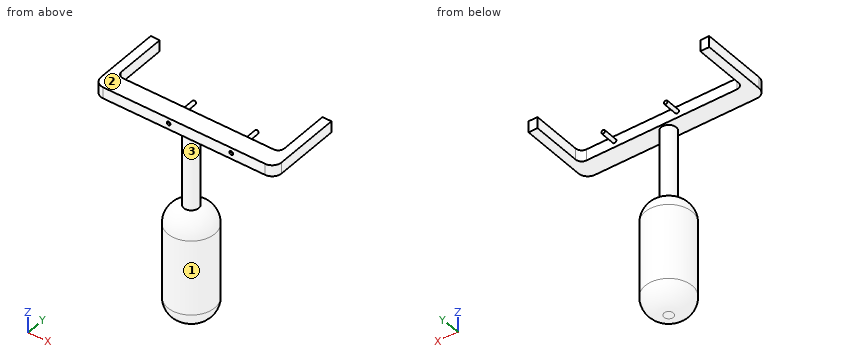
from build123d import *

# Parameters (mm, degrees)
F1_DEPTH  = 6
F2_R      = 3.25
F3_R      = 5
F4_R      = 1
F5_DEPTH  = 10
F6_R      = 4
F7_DEPTH  = 40
F8_R      = 12.5
F8_R_2    = 4
F9_DEPTH  = 60
F12_R     = 1
F13_DEPTH = 17


# Not quite as in the source:
# - a fillet or chamfer that OpenCascade refuses, or shapes differently, is made with other operations: its cross-section is extruded or revolved along the edge and cut away or added


with BuildPart() as f1:
    # F0 (on Top) → F1 (new body)
    with BuildSketch(Plane.XY):
        Polygon((-48, -5), (-48, -45), (48, -45), (48, -5), (43.25, -5), (43.25, -35), (-43.25, -35), (-43.25, -5), align=None)
    extrude(amount=F1_DEPTH)

    # F2
    f2_edges = [f1.edges().sort_by_distance(p)[0] for p in [
        (-43.25, -35, 3),
        (43.25, -35, 3),
    ]]
    fillet(f2_edges, radius=F2_R)

    # F3
    f3_edges = [f1.edges().sort_by_distance(p)[0] for p in [
        (48, -45, 3),
        (-48, -45, 3),
    ]]
    fillet(f3_edges, radius=F3_R)

    # F4 (on face) → F5 (cut)
    with BuildSketch(Plane.XZ.offset(45)):
        with Locations((-8.25, 3.2)):
            Circle(F4_R)
        with Locations((25, 3.2)):
            Circle(F4_R)
    extrude(amount=-F5_DEPTH, mode=Mode.SUBTRACT)

    # F6 (on face) → F7 (join)
    with BuildSketch(Plane(origin=(0, 0, 0), x_dir=(1, 0, 0), z_dir=(0, 0, -1))):
        with Locations((0, 40)):
            Circle(F6_R)
    extrude(amount=F7_DEPTH)

    # F8 (on face) → F9 (join)
    with BuildSketch(Plane(origin=(0, 0, -40), x_dir=(1, 0, 0), z_dir=(0, 0, -1))):
        with Locations((0, 40)):
            Circle(F8_R)
        with Locations((0, 40)):
            Circle(F8_R_2, mode=Mode.SUBTRACT)
        with Locations((0, 40)):
            Circle(F8_R_2)
    extrude(amount=F9_DEPTH)

    # F10: fillet of radius 10 on 2 edges, made by hand

    # F10_s1 → F10_t2 (revolve, cut)
    with BuildSketch(Plane.XZ.offset(40)):
        with BuildLine():
            ThreePointArc((12.5, -90), (9.5710678119, -97.0710678119), (2.5, -100))
            Line((2.5, -100), (12.5, -100))
            Line((12.5, -100), (12.5, -90))
        make_face()
    revolve(axis=Axis((0, -40, -100), (0, 0, -1)), mode=Mode.SUBTRACT)

    # F10_s3 → F10_t4 (revolve, cut)
    with BuildSketch(Plane.XZ.offset(40)):
        with BuildLine():
            ThreePointArc((12.5, -49.8868599666), (10.0828754441, -43.3676575614), (4, -40))
            Line((4, -40), (12.5, -40))
            Line((12.5, -40), (12.5, -49.8868599666))
        make_face()
    revolve(axis=Axis((0, -40, -40), (0, 0, -1)), mode=Mode.SUBTRACT)

    # F12 (on offset) → F13 (join)
    with BuildSketch(Plane.XZ.offset(44)):
        with Locations((-8.25, 3.2)):
            Circle(F12_R)
        with Locations((25, 3.2)):
            Circle(F12_R)
    extrude(amount=-F13_DEPTH)


solid = f1.part
Geometry check sheet. Reference: the model listing, model coordinates, mm. Face numbers are marked on the shaded views. Coordinates: 2 decimals unless noted, no trailing zeros. Order: outer loops, then holes, each group sorted by start corner. A loop starts at its lowest first (then second) coordinate and runs counter-clockwise, first axis right, second up. Notation, with made-up numbers: (62.5, 88.25) -> (104.5, 88.25) arc R17 ccw to (104.5, 97.25) -> close; hole circle Ø3 at (-17.5, -13.5). An arc over 180 degrees is marked (long way). Use a Markdown table: item, result. Add a question column.
1. Cross-section at A-A (y = -15). Enter the section's corners in (x, z).
2. Go/stop test with flat-tipped pins: pin 1 Ø0.6 at (x, z) = (-8, 3) entering from -Y; pin 2 Ø10 at (y, z) = (-25, -80.5) entering from +X; pin 3 Ø8 at (y, z) = (-45, -44) entering from +X; pin 4 Ø20 at (x, y) = (16.5, -16.5) entering from -Z. Record where each tip stops, or that it passes through.
3. Material ranges on L1, parallel to X at y = -14, z = 1; L2, parallel to X at y = -36.5, z = -12; L3, parallel to X at y = -35, z = -91.5, recorded low to high.
4. Mould release check, pull along Z, two halves, no side actions. Record for the marked faces 1, 2 and 3: pulls with the +Z half, pulls with the -Z half, needs draft (parallel to the pull), parting line crosses it, or undercut.
5. Cross-section at B-B (x = -14). Enter the section's corners in (y, z), and give its area (3 significant figures).
6. Cross-section at D-D (y = -30.5). Give the number of separate pieces and of enclosed holes in the cut face, and give its area (3 significant figures).
7. Cross-section at C-C (z = -22). Enter the section's corners in (x, y).
Filled sheet:
| question | item | result |
|---|---|---|
| 1 | outline | (-48, 0) -> (-43.25, 0) -> (-43.25, 6) -> (-48, 6) -> close; (43.25, 0) -> (48, 0) -> (48, 6) -> (43.25, 6) -> close |
| 2 | pin 1 | y = -44 |
| 2 | pin 2 | x = 7.5 |
| 2 | pin 3 | x = 11.85 |
| 2 | pin 4 | through |
| 3 | L1 | -48 to -43.25, 43.25 to 48 |
| 3 | L2 | -1.94 to 1.94 |
| 3 | L3 | -11.33 to 11.33 |
| 4 | face 1 | needs draft |
| 4 | face 2 | pulls with the +Z half |
| 4 | face 3 | undercut |
| 5 | outline | (-45, 0) -> (-35, 0) -> (-35, 6) -> (-45, 6) -> close |
| 5 | area | 60.0 mm2 |
| 6 | separate pieces | 5 |
| 6 | enclosed holes | 0 |
| 6 | area | 898 mm2 |
| 7 | outline | circle Ø8 at (0, -40) |
